```python
from build123d import *

# Parameters (mm, degrees)
M8_CLEARANCE_HOLE1_D     = 10
M8_CLEARANCE_HOLE1_DEPTH = 8.5
SKETCH4_R                = 6
CUT_EXTRUDE1_DEPTH       = 10


with BuildPart() as part:
    # Sketch1 → Revolve1 (revolve)
    with BuildSketch(Plane.XY):
        Polygon((-2.865, 4.25), (-2.865, 17.75), (0, 17.75), (0, 13.75), (5.635, 13.75), (5.635, 10.25), (0, 10.25), (0, 4.25), align=None)
    revolve(axis=Axis((-29.387999347, 0, 0), (1, 0, 0)))

    # M8 Clearance Hole1
    with Locations(Plane.ZY.offset(2.865)):
        with Locations((0, 0)):
            Hole(M8_CLEARANCE_HOLE1_D / 2, depth=M8_CLEARANCE_HOLE1_DEPTH)

    # Sketch4 → Cut-Extrude1 (cut)
    with BuildSketch(Plane.ZY.offset(2.865)):
        with Locations((-20.32, 0)):
            Circle(SKETCH4_R)
        with Locations((20.32, 0)):
            Circle(SKETCH4_R)
    extrude(amount=-CUT_EXTRUDE1_DEPTH, mode=Mode.SUBTRACT)


solid = part.part
```
Geometry check sheet. Reference: the model listing, model coordinates, mm. A direction names the side the tool comes from. Give positions to 0.01 mm unless a question says otherwise; leave off trailing zeros. Order: outer loops, then holes, each group sorted by start corner. A loop starts at its lowest first (then second) coordinate and runs counter-clockwise, first axis right, second up. Notation, with made-up numbers: (6.25, 59) - (35.25, 59) arc R14 ccw to (35.25, 69) - close; hole circle Ø9 at (49, -32.75). An arc over 180 degrees is marked (long way). Answer in a Markdown table with one row per item. Add a question column.
Q1. Tool access check on faces 5 (the cylindrical face through (2.857, -2.981, -13.423)), 6 (the flat face through (-2.865, -4, -4)). Record the directions out of +Z, -Z, +X, -X, +Y, -Y that give a thin tool (end or side, any length) a straight path to the whole face; none if there is none.
Q2. Cross-section at C-C, the plane x = -1. Enter the section's corners in (y, z), then the cut area to 3 significant figures.
Q3. Gauge pin test, flat ends, axial feed: pin 1 (2 mm diameter, centred on x = 0, z = -10, fed in from +Y); pin 2 (1.5 mm diameter, centred on x = 3, y = -5, fed in from +Z); pin 3 (1 mm diameter, centred on x = 4.5, y = 8, fed in from +Z). Record the tip position at first contact, or that the pin passes through.
Q4. Cross-section at A-A, the plane y = 0. Enter the section's corners in (x, z) (3 decimals).
Q5. Material ranges on probe 1 along Z at (x, y) = (4, 0); probe 2 along Y at (x, z) = (4, -3); probe 3 along Y at (x, z) = (-2, -15), recorded low to high. Write a range as from..to.
Q6. Cross-section at B-B, the plane z = 0. Enter the section's corners in (x, y) (3 decimals), then the cut area to 3 significant figures.
Q7. Cross-section at D-D, the plane z = 8.5. Enter the section's corners in (x, y) (3 decimals), then the cut area to 3 significant figures.
Q8. Mould release check, pull along Y, two halves, no side actions. Record for faces 1 (the cylindrical face through (-1.412, -17.747, 0.319)), 2 (the flat face through (5.635, -5.2, -9.1)), 3 (the cylindrical face through (-1.45, -0.08, -14.32)), 4 (the cylindrical face through (-1.45, 0.08, 14.32)): pulls with the +Y half, pulls with the -Y half, needs draft (parallel to the pull), parting line crosses it, or undercut.
Check values:
| question | item | result |
|---|---|---|
| 1 | face 5 | +X |
| 1 | face 6 | +Z, -Z, -X, +Y, -Y |
| 2 | outline | (-5.02, -17.03) arc R6 cw to (5.02, -17.03) arc R17.75 ccw to (5.02, 17.03) arc R6 cw to (-5.02, 17.03) arc R17.75 ccw to start; hole circle Ø10 at (0, 0) |
| 2 | area | 863 mm^2 |
| 3 | pin 1 | stops at y = 15.3 |
| 3 | pin 2 | stops at z = 13.08 |
| 3 | pin 3 | stops at z = 11.52 |
| 4 | outline | (-2.865, -14.32) - (0, -14.32) - (0, -13.75) - (5.635, -13.75) - (5.635, -10.25) - (0, -10.25) - (0, -5) - (-2.865, -5) - close; (-2.865, 5) - (0, 5) - (0, 10.25) - (5.635, 10.25) - (5.635, 13.75) - (0, 13.75) - (0, 14.32) - (-2.865, 14.32) - close |
| 5 | probe 1 | z = -13.75..-10.25, 10.25..13.75 |
| 5 | probe 2 | y = -13.42..-9.8, 9.8..13.42 |
| 5 | probe 3 | y = -9.49..-2.77, 2.77..9.49 |
| 6 | outline | (-2.865, -17.75) - (0, -17.75) - (0, -13.75) - (5.635, -13.75) - (5.635, -10.25) - (0, -10.25) - (0, -5) - (-2.865, -5) - close; (-2.865, 5) - (0, 5) - (0, 10.25) - (5.635, 10.25) - (5.635, 13.75) - (0, 13.75) - (0, 17.75) - (-2.865, 17.75) - close |
| 6 | area | 113 mm^2 |
| 7 | outline | (-2.865, -15.582) - (0, -15.582) - (0, -10.808) - (5.635, -10.808) - (5.635, -5.728) - (0, -5.728) - (0, 5.728) - (5.635, 5.728) - (5.635, 10.808) - (0, 10.808) - (0, 15.582) - (-2.865, 15.582) - close |
| 7 | area | 147 mm^2 |
| 8 | face 1 | pulls with the -Y half |
| 8 | face 2 | needs draft |
| 8 | face 3 | undercut |
| 8 | face 4 | undercut |
